from build123d import *

# Parameters (mm, degrees)
F0_W     = 44.45
F0_H     = 508
F1_DEPTH = 6.35
F3_D     = 5.1054
F4_R     = 3
F5_DEPTH = 6.35
F6_R     = 4.7625
F7_DEPTH = 6.35


with BuildPart() as f1:
    # F0 (on Top) → F1 (new body)
    with BuildSketch(Plane.XY):
        Rectangle(F0_W, F0_H)
    extrude(amount=F1_DEPTH)

    # F3 (through all)
    with Locations(Plane.XY.offset(6.35)):
        with Locations((-15.875, -215.9), (15.875, -215.9), (15.875, -161.925), (-15.875, -161.925), (-15.875, -107.95), (15.875, -107.95), (15.875, -53.975), (-15.875, -53.975), (-15.875, 0), (15.875, 0), (15.875, 53.975), (-15.875, 53.975), (-15.875, 107.95), (15.875, 107.95), (-15.875, 161.925), (15.875, 161.925), (15.875, 215.9), (-15.875, 215.9)):
            Hole(F3_D / 2)

    # F4 (on face) → F5 (cut, through all)
    with BuildSketch(Plane.XY.offset(6.35)):
        with Locations((0, -239)):
            Circle(F4_R)
        with Locations((0, 239)):
            Circle(F4_R)
    extrude(amount=-F5_DEPTH, mode=Mode.SUBTRACT)

    # F6 (on face) → F7 (cut, through all)
    with BuildSketch(Plane.XY.offset(6.35)):
        Circle(F6_R)
    extrude(amount=-F7_DEPTH, mode=Mode.SUBTRACT)


solid = f1.part
Part model, mm, in its own coordinate system. Give positions to 0.01 mm unless a question says otherwise; leave off trailing zeros. Use one line per item in the form item = value.
(1) Drill centre lines: line 1 (Y direction, x = 0, z = 2.5); line 2 (Y direction, x = 0.5, z = 4); line 3 (X direction, y = -215.9, z = 1.75) (3 decimals). Where is each one in solid material? Low to high. Write a range as from..to.
Solution:
line_1 = -254..-242, -236..-4.76, 4.76..236, 242..254
line_2 = -254..-241.96, -236.04..-4.74, 4.74..236.04, 241.96..254
line_3 = -22.225..-18.428, -13.322..13.322, 18.428..22.225
(2) Flat gauge pin, fed straight in: P1, Ø4, axis at x = -15.875, y = 0, coming from the -Z side. Where does the tip first touch, or does it go through?
Solution:
P1 = through
(3) Pull direction Y, two halves, no side cores. Call faces 1 (the face through (-5, 4, 6.35)), 2 (the face through (-3.78, -2.9, 3.22)): +Y half, -Y half, draft (parallel to the pull), parting line (faces both ways), or undercut.
Solution:
face_1 = draft
face_2 = undercut
(4) Saw through at A-A (z = 1.5). Count the separate pieces of the cut face and the enclosed holes in it, then the cut area to 3 significant figures.
Solution:
separate_pieces = 1
enclosed_holes = 21
area = 22,100 mm²
